Read the model definition and answer for the solid it produces. Units are mm, in the model's axes. Coordinates: 2 decimals unless noted, no trailing zeros. Write each loop counter-clockwise with the first axis right and the second up, starting at its lowest first coordinate (ties: lowest second). Pieces come first, ordered by that corner, then holes.
1) The part is cut by section C-C (x = 86). Determine the outline of the cut face in (y, z).
2) The part is cut by section B-B (y = -6.5). Determine the outline of the cut face in (x, z), then the cut area to 3 significant figures.
3) Find the intervals of material crossed by line 1 (X direction, y = 15.5, z = 0.65); line 2 (Y direction, x = -30, z = 1.15); line 3 (X direction, y = 78.5, z = 0.45), in increasing order.
4) The part is cut by section A-A (z = 1.55). Give the number of separate pieces and of enclosed holes in the cut face, then the cut area to 3 significant figures.
5) Each of these flat-tipped pins is pushed along its axis until it touches: pin 1 Ø1 at (y, z) = (-7.5, 1.5) entering from +X; pin 2 Ø4 at (x, y) = (-30, 15.5) entering from -Z; pin 3 Ø1 at (y, z) = (-12, 1) entering from -X; pin 4 Ø0.6 at (x, z) = (89.5, 1) entering from -Y. Where does it stop, or does it pass through?
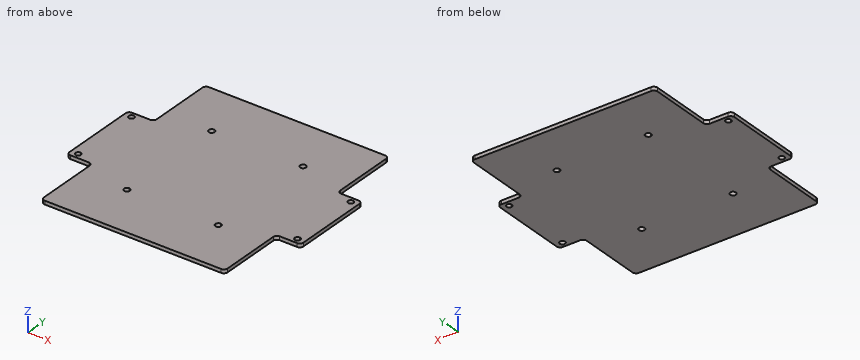
from build123d import *

# Parameters (mm, degrees)
SKETCH_1_W               = 60
SKETCH_1_H               = 70
SKETCH_1_R               = 1.5
EXTRUDE_1_DEPTH          = 2
SKETCH_2_W               = 34
SKETCH_2_H               = 45
EXTRUDE_2_DEPTH          = 2
CUT_EXTRUDE_1_DEPTH      = 1
CUT_EXTRUDE_1_DEPTH_BACK = 118.217746097
FILLET_1_R               = 2
CUT_EXTRUDE_2_DEPTH      = 118.217746097
PATTERN_LINEAR_1_COUNT   = 4
PATTERN_LINEAR_1_PITCH   = 14
SKETCH_6_W               = 100.507986439
SKETCH_6_H               = 120
EXTRUDE_3_DEPTH          = 2
CUT_EXTRUDE_3_DEPTH      = 3
FILLET_2_R               = 2


with BuildPart() as part:
    # Sketch 1 → Extrude 1 (new body)
    with BuildSketch(Plane.XY):
        with Locations((30, 35)):
            Rectangle(SKETCH_1_W, SKETCH_1_H)
        with Locations((5, 66)):
            Circle(SKETCH_1_R, mode=Mode.SUBTRACT)
        with Locations((55, 66)):
            Circle(SKETCH_1_R, mode=Mode.SUBTRACT)
        with Locations((5, 4)):
            Circle(SKETCH_1_R, mode=Mode.SUBTRACT)
        with Locations((55, 4)):
            Circle(SKETCH_1_R, mode=Mode.SUBTRACT)
    extrude(amount=EXTRUDE_1_DEPTH)

    # Sketch 2 → Extrude 2 (add)
    with BuildSketch(Plane.XY.offset(2)):
        with Locations((77, 35)):
            Rectangle(SKETCH_2_W, SKETCH_2_H)
    extrude_2 = extrude(amount=-EXTRUDE_2_DEPTH)

    # Mirror 1: Extrude 2 across plane
    add(extrude_2.mirror(Plane(origin=(30, 0, 0), x_dir=(0, 0, 1), z_dir=(1, 0, 0))))

    # Sketch 3 → Cut-Extrude 1 (cut, two sides: drawn at the far end of the back side and taken through both)
    with BuildSketch(Plane.XY.offset(2).offset(-CUT_EXTRUDE_1_DEPTH_BACK)):
        with BuildLine():
            Line((-30, 53), (-30, 54.5))
            Line((-30, 54.5), (-28.5, 54.5))
            ThreePointArc((-28.5, 54.5), (-31.060660172, 55.560660172), (-30, 53))
        make_face()
        with BuildLine():
            Line((-28.5, 54.5), (-30, 54.5))
            Line((-30, 54.5), (-30, 53))
            ThreePointArc((-30, 53), (-28.939339828, 53.439339828), (-28.5, 54.5))
        make_face()
        with BuildLine():
            ThreePointArc((-28.5, 15.5), (-28.939339828, 16.560660172), (-30, 17))
            Line((-30, 17), (-30, 15.5))
            Line((-30, 15.5), (-28.5, 15.5))
        make_face()
        with BuildLine():
            Line((-30, 15.5), (-30, 17))
            ThreePointArc((-30, 17), (-31.060660172, 14.439339828), (-28.5, 15.5))
            Line((-28.5, 15.5), (-30, 15.5))
        make_face()
        with BuildLine():
            ThreePointArc((91.5, 54.5), (90, 56), (88.5, 54.5))
            Line((88.5, 54.5), (90, 54.5))
            Line((90, 54.5), (90, 53))
            ThreePointArc((90, 53), (91.060660172, 53.439339828), (91.5, 54.5))
        make_face()
        with BuildLine():
            Line((90, 54.5), (88.5, 54.5))
            ThreePointArc((88.5, 54.5), (88.939339828, 53.439339828), (90, 53))
            Line((90, 53), (90, 54.5))
        make_face()
        with BuildLine():
            ThreePointArc((91.5, 15.5), (91.060660172, 16.560660172), (90, 17))
            Line((90, 17), (90, 15.5))
            Line((90, 15.5), (88.5, 15.5))
            ThreePointArc((88.5, 15.5), (90, 14), (91.5, 15.5))
        make_face()
        with BuildLine():
            Line((90, 15.5), (90, 17))
            ThreePointArc((90, 17), (88.939339828, 16.560660172), (88.5, 15.5))
            Line((88.5, 15.5), (90, 15.5))
        make_face()
    extrude(amount=CUT_EXTRUDE_1_DEPTH + CUT_EXTRUDE_1_DEPTH_BACK, mode=Mode.SUBTRACT)

    # Fillet 1
    fillet_1_edges = [part.edges().sort_by_distance(p)[0] for p in [
        (0, 0, 1),
        (0, 70, 1),
        (60, 70, 1),
        (60, 0, 1),
        (60, 12.5, 1),
        (60, 57.5, 1),
        (94, 57.5, 1),
        (94, 12.5, 1),
        (0, 57.5, 1),
        (0, 12.5, 1),
        (-34, 12.5, 1),
        (-34, 57.5, 1),
    ]]
    fillet(fillet_1_edges, radius=FILLET_1_R)

    # Sketch 4 → Cut-Extrude 2 (cut, through all)
    with BuildSketch(Plane.XY.offset(2)):
        with BuildLine():
            Line((15, 55), (15, 15))
            ThreePointArc((15, 15), (11, 11), (7, 15))
            Line((7, 15), (7, 55))
            ThreePointArc((7, 55), (11, 59), (15, 55))
        make_face()
    cut_extrude_2 = extrude(amount=-CUT_EXTRUDE_2_DEPTH, mode=Mode.SUBTRACT)

    # Pattern Linear 1: Cut-Extrude 2 ×4
    with Locations(*[(i * PATTERN_LINEAR_1_PITCH, 0, 0) for i in range(1, PATTERN_LINEAR_1_COUNT)]):
        add(cut_extrude_2, mode=Mode.SUBTRACT)

    # Sketch 6 → Extrude 3 (add)
    with BuildSketch(Plane.XY.offset(2)):
        with Locations((30.25399322, 35)):
            Rectangle(SKETCH_6_W, SKETCH_6_H)
    extrude(amount=-EXTRUDE_3_DEPTH)

    # Sketch 7 → Cut-Extrude 3 (cut)
    with BuildSketch(Plane.XY.offset(2)):
        with BuildLine():
            ThreePointArc((6.85399322, 66), (4.12262237, 67.13137085), (5.25399322, 64.4))
            Line((5.25399322, 64.4), (5.25399322, 66))
            Line((5.25399322, 66), (6.85399322, 66))
        make_face()
        with BuildLine():
            Line((5.25399322, 66), (5.25399322, 64.4))
            ThreePointArc((5.25399322, 64.4), (6.38536407, 64.86862915), (6.85399322, 66))
            Line((6.85399322, 66), (5.25399322, 66))
        make_face()
        with BuildLine():
            ThreePointArc((53.65399322, 66), (54.12262237, 64.86862915), (55.25399322, 64.4))
            Line((55.25399322, 64.4), (55.25399322, 66))
            Line((55.25399322, 66), (53.65399322, 66))
        make_face()
        with BuildLine():
            Line((55.25399322, 66), (55.25399322, 64.4))
            ThreePointArc((55.25399322, 64.4), (56.38536407, 64.86862915), (56.85399322, 66))
            ThreePointArc((56.85399322, 66), (55.25399322, 67.6), (53.65399322, 66))
            Line((53.65399322, 66), (55.25399322, 66))
        make_face()
        with BuildLine():
            ThreePointArc((5.25399322, 5.6), (4.12262237, 2.86862915), (6.85399322, 4))
            Line((6.85399322, 4), (5.25399322, 4))
            Line((5.25399322, 4), (5.25399322, 5.6))
        make_face()
        with BuildLine():
            Line((5.25399322, 4), (6.85399322, 4))
            ThreePointArc((6.85399322, 4), (6.38536407, 5.13137085), (5.25399322, 5.6))
            Line((5.25399322, 5.6), (5.25399322, 4))
        make_face()
        with BuildLine():
            ThreePointArc((55.25399322, 5.6), (54.12262237, 5.13137085), (53.65399322, 4))
            Line((53.65399322, 4), (55.25399322, 4))
            Line((55.25399322, 4), (55.25399322, 5.6))
        make_face()
        with BuildLine():
            Line((55.25399322, 4), (53.65399322, 4))
            ThreePointArc((53.65399322, 4), (55.25399322, 2.4), (56.85399322, 4))
            ThreePointArc((56.85399322, 4), (56.38536407, 5.13137085), (55.25399322, 5.6))
            Line((55.25399322, 5.6), (55.25399322, 4))
        make_face()
    extrude(amount=-CUT_EXTRUDE_3_DEPTH, mode=Mode.SUBTRACT)

    # Fillet 2
    fillet_2_edges = [part.edges().sort_by_distance(p)[0] for p in [
        (-20, 57.5, 1),
        (80.507986439, 12.5, 1),
        (80.507986439, 57.5, 1),
        (80.507986439, 95, 1),
        (-20, -25, 1),
        (-20, 95, 1),
        (80.507986439, -25, 1),
        (-20, 12.5, 1),
    ]]
    fillet(fillet_2_edges, radius=FILLET_2_R)


solid = part.part
Reported:
1. outline: (12.5, 0) - (57.5, 0) - (57.5, 2) - (12.5, 2) - close
2. outline: (-20, 0) - (80.51, 0) - (80.51, 2) - (-20, 2) - close
2. area: 201 mm2
3. line 1: x = -34 to -31.5, -28.5 to 88.5, 91.5 to 94
3. line 2: y = 12.5 to 14, 17 to 53, 56 to 57.5
3. line 3: x = -20 to 80.51
4. separate pieces: 1
4. enclosed holes: 8
4. area: 13,200 mm2
5. pin 1: stops at x = 80.51
5. pin 2: stops at z = 0
5. pin 3: stops at x = -20
5. pin 4: stops at y = 12.5
